Read the model definition and answer for the solid it produces. Units are mm, in the model's axes. A direction names the side the tool comes from. Give positions to 0.01 mm unless a question says otherwise; leave off trailing zeros. Order: outer loops, then holes, each group sorted by start corner. A loop starts at its lowest first (then second) coordinate and runs counter-clockwise, first axis right, second up.
Item 1: Given pin 1 Ø1.1 at (x, y) = (4, 0) entering from +Z; pin 2 Ø1.8 at (x, y) = (-6, 0.5) entering from -Z; pin 3 Ø2 at (x, y) = (0, 0.5) entering from +Z; pin 4 Ø4 at (x, y) = (0.5, 1) entering from +Z, each flat-ended and moving along its own axis, determine where each tip first touches the part or whether it passes through.
Item 2: Which of the six approach directions +Z, -Z, +X, -X, +Y, -Y give full straight-line access (tool end or side, diameter ignored) to faces 1 (the face through (-9.01, 0.7, 3.41)), 2 (the face through (-10.171, -1.045, -2.26)), 3 (the face through (-9.01, 0.7, 5.31))?
Item 3: A cutting plane is placed at A-A (z = -1). Write down the section's boundary in (x, y), plus the area to 3 significant figures.
Item 4: The mould has two halves that part along X. Classify faces 4 (the face through (-10.7, 0, 2)), 5 (the face through (11.4, 0, 0)), 6 (the face through (-0.2, -2.3, -3)): +X half, -X half, draft (parallel to the pull), parting line (faces both ways), or undercut.
Item 5: Find the intervals of material crossed by line 1 along X through (y, z) = (1.5, -0.5); line 2 along X through (y, z) = (0.5, -2.25); line 3 along Y through (x, z) = (-3, -1.25), in increasing order.
Item 6: A cutting plane is placed at B-B (x = -1.25). Write down the section's boundary in (y, z), plus the area to 3 significant figures.
Item 7: A cutting plane is placed at C-C (z = 0.5). Write down the section's boundary in (x, y), plus the area to 3 significant figures.
Item 8: A cutting plane is placed at D-D (x = 8). Write down the section's boundary in (y, z).
Autodesk Inventor part; units mm, degrees
ref_plane "Work Plane1" through (-8.1, 0, 4.8) normal (0, 0, 1) x (1, 0, 0)
ref_plane "Work Plane2" through (-11.4, 0, 3) normal (0, -1, 0) x (1, 0, 0)
ref_plane "YZ Plane" through (0, 0, 0) normal (1, 0, 0) x (0, 1, 0)
sketch "Sketch1" plane through (0, 0, 0) normal (0, 0, 1) x (1, 0, 0)
  line L0 (-11.4, -3.5) -> (11.4, -3.5)
  line L1 (11.4, -3.5) -> (11.4, 3.5)
  line L2 (11.4, 3.5) -> (-11.4, 3.5)
  line L3 (-11.4, 3.5) -> (-11.4, -3.5)
  line L4 (-11.4, -3.5) -> (11.4, 3.5) construction
  line L5 (11.4, -3.5) -> (-11.4, 3.5) construction
  point P0 (0, 0)
  dimension "d0" = 22.8
  dimension "d1" = 7
extrude "Extrusion1" add sketch "Sketch1" along normal mid plane 6
sketch "Sketch2" plane through (0, 0, 3) normal (0, 0, 1) x (1, 0, 0)
  line L0 (-5, 2.1) -> (-0.5, 2.1)
  line L1 (-0.5, 2.1) -> (-0.5, -2.1)
  line L2 (-0.5, -2.1) -> (-5, -2.1)
  line L3 (-5, -2.1) -> (-5, 2.1)
  line L4 (-5, 2.1) -> (-0.5, -2.1) construction
  line L5 (-0.5, 2.1) -> (-5, -2.1) construction
  line L6 (-11.4, 3.5) -> (-11.4, -3.5)
  line L7 (-2.75, 0) -> (-11.4, 0) construction
  point P0 (0, 0)
  dimension "d4" = 4.2
  dimension "d5" = 4.5
  dimension "d6" = 6.4
extrude "Extrusion2" cut sketch "Sketch2" against normal through all
sketch "Sketch3" plane through (0, 0, 3) normal (0, 0, 1) x (1, 0, 0)
  line L0 (-5, -2.1) -> (-5, 2.1)
  line L1 (-5, 2.1) -> (-0.5, 2.1)
  line L2 (-0.5, 2.1) -> (-0.5, -2.1)
  line L3 (-0.5, -2.1) -> (-5, -2.1)
  line L4 (-11.4, -3.5) -> (11.4, -3.5)
  line L5 (11.4, -3.5) -> (11.4, 3.5)
  line L6 (11.4, 3.5) -> (-11.4, 3.5)
  line L7 (-11.4, 3.5) -> (-11.4, -3.5)
  line L8 (-10.7, -2.6) -> (10.5, -2.6)
  line L9 (10.5, -2.6) -> (10.5, 2.6)
  line L10 (10.5, 2.6) -> (-10.7, 2.6)
  line L11 (-10.7, 2.6) -> (-10.7, -2.6)
  line L12 (-10.7, -2.6) -> (10.5, 2.6) construction
  line L13 (10.5, -2.6) -> (-10.7, 2.6) construction
  dimension "d11" = 0.7
  dimension "d12" = 0.9
  dimension "d13" = 5.2
  dimension "d14" = 21.2
extrude "Extrusion3" cut sketch "Sketch3" against normal blind 1.5 contours L11 L10 L9 L8
sketch "Sketch4" plane through (0, 0, -3) normal (0, 0, -1) x (-1, 0, 0)
  line L0 (-2.6, -2.1) -> (5, -2.1)
  line L1 (5, -2.1) -> (5, 2.1)
  line L2 (5, 2.1) -> (-2.6, 2.1)
  line L3 (-2.6, 2.1) -> (-2.6, -2.1)
  line L4 (-2.6, -2.1) -> (5, 2.1) construction
  line L5 (5, -2.1) -> (-2.6, 2.1) construction
  line L6 (5, 2.1) -> (5, -2.1)
  line L7 (5, -2.1) -> (0.5, -2.1)
  line L8 (0.5, -2.1) -> (0.5, 2.1)
  line L9 (0.5, 2.1) -> (5, 2.1)
  line L10 (-11.4, -3.5) -> (11.4, -3.5)
  line L11 (11.4, -3.5) -> (11.4, 3.5)
  line L12 (11.4, 3.5) -> (-11.4, 3.5)
  line L13 (-11.4, 3.5) -> (-11.4, -3.5)
  line L14 (0.5, 2.1) -> (5, 2.1)
  line L15 (5, -2.1) -> (0.5, -2.1)
  line L16 (5, 2.1) -> (5, -2.1)
  point P0 (0, 0)
  point P1 (1.2, 0)
  dimension "d17" = 14
extrude "Extrusion4" cut sketch "Sketch4" against normal blind 2.9 contours L3 L2 L8 L0 | L8 L2 L1 L0
sketch "Sketch5" plane through (0, 0, -3) normal (0, 0, -1) x (-1, 0, 0)
  line L0 (6.4, -2.1) -> (-6.5, -2.1)
  line L1 (-6.5, -2.1) -> (-6.5, 2.1)
  line L2 (-6.5, 2.1) -> (6.4, 2.1)
  line L3 (6.4, 2.1) -> (6.4, -2.1)
  line L4 (6.4, -2.1) -> (-6.5, 2.1) construction
  line L5 (-6.5, -2.1) -> (6.4, 2.1) construction
  line L6 (-2.6, 2.1) -> (5, 2.1)
  line L7 (5, -2.1) -> (-2.6, -2.1)
  line L8 (11.4, -3.5) -> (11.4, 3.5)
  point P0 (0, 0)
  point P1 (-0.05, 0)
  dimension "d20" = 12.9
  dimension "d21" = 5
extrude "Extrusion5" cut sketch "Sketch5" against normal blind 2.4
sketch "Sketch6" plane through (0, 0, -3) normal (0, 0, -1) x (-1, 0, 0)
  line L0 (-6.5, 2.1) -> (6.4, 2.1)
  line L1 (6.4, 2.1) -> (6.4, -2.1)
  line L2 (6.4, -2.1) -> (-6.5, -2.1)
  line L3 (-6.5, -2.1) -> (-6.5, 2.1)
  line L4 (-11.4, -3.5) -> (11.4, -3.5)
  line L5 (11.4, -3.5) -> (11.4, 3.5)
  line L6 (11.4, 3.5) -> (-11.4, 3.5)
  line L7 (-11.4, 3.5) -> (-11.4, -3.5)
  point P0 (0, 0)
hole "Hole1" at (-6.4, 2.1, -3) at (-6.4, -2.1, -3) at (6.5, -2.1, -3) at (6.5, 2.1, -3) direction (0, 0, 1) diameter 0.5 depth 2.4
sketch "Sketch7" plane through (0, 0, -3) normal (0, 0, -1) x (-1, 0, 0)
  line L0 (-11.4, -3.5) -> (11.4, -3.5)
  line L1 (11.4, -3.5) -> (11.4, 3.5)
  line L2 (11.4, 3.5) -> (-11.4, 3.5)
  line L3 (-11.4, 3.5) -> (-11.4, -3.5)
  arc A0 (-6.5, -1.85) -> (-6.25, -2.1) centre (-6.5, -2.1) ccw
  line L4 (-6.5, -1.85) -> (-6.5, 1.85)
  arc A1 (-6.25, 2.1) -> (-6.5, 1.85) centre (-6.5, 2.1) ccw
  line L5 (-6.25, 2.1) -> (6.15, 2.1)
  arc A2 (6.4, 1.85) -> (6.15, 2.1) centre (6.4, 2.1) ccw
  line L6 (6.4, 1.85) -> (6.4, -1.85)
  arc A3 (6.15, -2.1) -> (6.4, -1.85) centre (6.4, -2.1) ccw
  line L7 (6.15, -2.1) -> (-6.25, -2.1)
  line L8 (-6.5, -1.85) -> (-6.5, 1.85)
  line L9 (-11.4, 3.5) -> (-11.4, -3.5)
  line L10 (11.4, -3.5) -> (11.4, 3.5)
  line L11 (6.4, 1.85) -> (6.4, -1.85)
  arc A4 (9.4189, -0.0387) -> (6.4, 2.1) centre (6.4, -1.1) ccw
  arc A5 (8.4755, -0.3703) -> (6.4, 1.1) centre (6.4, -1.1) ccw
  arc A6 (9.4189, -0.0387) -> (11.4, -1.4422) centre (11.4, 0.6578) ccw
  arc A7 (8.4755, -0.3703) -> (11.4, -2.4422) centre (11.4, 0.6578) ccw
  line L12 (6.4, 1.1) -> (6.4, 2.1)
  line L13 (11.4, -2.4422) -> (11.4, -1.4422)
  line L14 (11.4, 3.5) -> (11.4, -3.5)
  point P0 (0, 0)
  dimension "d36" = 1
  dimension "d37" = 2.2
  dimension "d38" = 2.1
extrude "Extrusion7" cut sketch "Sketch7" against normal blind 1.5 contours A7 A5 L6 A2 A4 A6 L1 | A2 L12 A4
sketch "Sketch8" plane through (0, 0, -0.6) normal (0, 0, -1) x (-1, 0, 0)
  line L0 (11.4, 3.5) -> (-11.4, 3.5)
  line L1 (11.4, -3.5) -> (11.4, -2.4422)
  point P0 (0, 0)
  point P1 (-4, 0)
  dimension "d41" = 3.5
  dimension "d42" = 15.4
hole "Hole2" at (4, 0, -0.6) direction (0, 0, 1) diameter 1.181 end through all
sketch "Sketch9" plane through (0, 0, 1.5) normal (0, 0, 1) x (1, 0, 0)
  circle A0 centre (-8.1, 0) radius 1.15
  circle A1 centre (8, 0) radius 1.15
  line L0 (-8.1, 0) -> (8, 0) construction
  line L1 (11.4, 3.5) -> (-11.4, 3.5)
  line L2 (-11.4, 3.5) -> (-11.4, -3.5)
  point P0 (0, 0)
  dimension "d50" = 3.5
  dimension "d51" = 16.1
  dimension "d52" = 3.3
  dimension "d53" = 2.3
extrude "Extrusion8" add sketch "Sketch9" along normal blind 4.5
chamfer "Chamfer1" distance 0.3 angle 45 2 edges at (-9.25, 0, 6) (6.85, 0, 6)
ref_plane "Work Plane1" through (-8.1, 0, 4.8) normal (0, 0, 1) x (1, 0, 0)
sketch "Sketch10" plane through (-8.1, 0, 4.8) normal (0, 0, 1) x (1, 0, 0)
  circle A0 centre (0, 0) radius 1.15
  circle A1 centre (16.1, 0) radius 1.15
  circle A2 centre (0, 0) radius 1.2
  circle A3 centre (16.1, 0) radius 1.2
  point P0 (8.1, 0)
  dimension "d60" = 2.4
  dimension "d61" = 2.4
extrude "Extrusion9" add sketch "Sketch10" against normal blind 0.2
ref_plane "Work Plane2" through (-11.4, 0, 3) normal (0, -1, 0) x (1, 0, 0)
sketch "Sketch11" plane through (-11.4, 0, 3) normal (0, -1, 0) x (1, 0, 0)
  line L0 (4.45, 2.7) -> (2.15, 2.7)
  line L1 (4.45, 1.8) -> (2.15, 1.8)
  line L2 (2.1, 1.6) -> (4.5, 1.6)
  line L3 (2.1, 1.8) -> (4.5, 1.8)
  line L4 (2.15, 1.6) -> (4.45, 1.6)
  line L5 (2.15, -1.5) -> (4.45, -1.5)
  line L6 (20.55, 2.7) -> (18.25, 2.7)
  line L7 (20.55, 1.8) -> (18.25, 1.8)
  line L8 (18.2, 1.6) -> (20.6, 1.6)
  line L9 (18.2, 1.8) -> (20.6, 1.8)
  line L10 (18.25, 1.6) -> (20.55, 1.6)
  line L11 (18.25, -1.5) -> (20.55, -1.5)
  line L12 (2.1, 1.8) -> (4.5, 1.8)
  line L13 (2.1, 1.8) -> (2.15, 1.9374)
  line L14 (2.1, 1.6) -> (2.15, 1.55)
  line L15 (2.15, -1.5) -> (2.15, 1.6)
  line L16 (2.15, 1.8) -> (2.15, 2.7)
  line L17 (2.15, 1.9374) -> (2.15, 1.8)
  line L18 (2.1, 1.8) -> (2.15, 1.8)
  line L19 (2.15, 1.55) -> (2.15, 1.6)
  line L20 (2.1, 1.6) -> (4.5, 1.6)
  line L21 (2.1, 1.6) -> (2.15, 1.6)
  line L22 (2.45, 3) -> (4.15, 3)
  line L23 (3.3, 3) -> (3.3, 1.6)
  line L24 (2.15, 1.6) -> (4.45, 1.6)
  point P0 (11.4, -3)
  dimension "d68" = 20
  dimension "d69" = 45
revolve "Revolution1" add sketch "Sketch11" angle 360 about axis through (-8.1, 0, 6) along (0, 0, -1) contours L15 L14 L2 | L16 L3 L13
sketch "Sketch12" plane through (-11.4, 0, 3) normal (0, -1, 0) x (1, 0, 0)
  line L0 (18.25, 1.8) -> (18.25, 2.7)
  line L1 (18.2, 1.8) -> (20.6, 1.8)
  line L2 (18.2, 1.8) -> (18.2, 1.6)
  line L3 (18.25, -1.5) -> (18.25, 1.6)
  line L4 (18.2, 1.6) -> (20.6, 1.6)
  line L5 (20.6, 1.8) -> (20.6, 1.6)
  line L6 (20.55, 1.8) -> (20.55, 2.7)
  line L7 (20.55, -1.5) -> (20.55, 1.6)
  line L8 (18.2, 1.8) -> (18.25, 1.9374)
  line L9 (20.55, 1.8) -> (18.25, 1.8)
  line L10 (18.25, 1.8) -> (18.25, 1.9374)
  line L11 (18.25, 1.8) -> (18.2, 1.8)
  line L12 (18.25, 1.55) -> (18.2, 1.6)
  line L13 (18.25, 1.6) -> (20.55, 1.6)
  line L14 (18.25, 1.6) -> (18.2, 1.6)
  line L15 (18.25, 1.6) -> (18.25, 1.55)
  line L16 (18.55, 3) -> (20.25, 3)
  line L17 (19.4, 3) -> (19.4, 1.6)
  point P0 (11.4, -3)
  dimension "d71" = 70
  dimension "d72" = 45
revolve "Revolution2" add sketch "Sketch12" angle 360 about axis through (8, 0, 6) along (0, 0, -1) contours L1 L8 L0 | L4 L3 L12
fillet "Fillet1" radius 0.8 2 edges at (-9.25, 0, 1.5) (6.85, 0, 1.5)
properties part number "sipmHolder" material "ABS Plastic"
Response values:
1. pin 1: passes through
1. pin 2: stops at z = -3
1. pin 3: stops at z = 1.5
1. pin 4: stops at z = 3
2. face 1: none
2. face 2: -Z
2. face 3: +Z
3. outline: (-11.4, -3.5) - (11.4, -3.5) - (11.4, 3.5) - (-11.4, 3.5) - close; hole (-6.4, -1.85) arc R0.25 ccw (long way) to (-6.15, -2.1) - (6.25, -2.1) arc R0.25 ccw (long way) to (6.5, -1.85) - (6.5, 1.85) arc R0.25 ccw (long way) to (6.25, 2.1) - (-6.15, 2.1) arc R0.25 ccw (long way) to (-6.4, 1.85) - close
3. area: 105 mm2
4. face 4: undercut
4. face 5: +X half
4. face 6: draft
5. line 1: x = -11.4 to -5, 2.6 to 11.4
5. line 2: x = -11.4 to -9.17, -7.91 to -6.4, 6.5 to 11.4
5. line 3: y = -3.5 to -2.1, 2.1 to 3.5
6. outline: (-3.5, -3) - (-2.1, -3) - (-2.1, 1.5) - (-2.6, 1.5) - (-2.6, 3) - (-3.5, 3) - close; (2.1, -3) - (3.5, -3) - (3.5, 3) - (2.6, 3) - (2.6, 1.5) - (2.1, 1.5) - close
6. area: 15.3 mm2
7. outline: (-11.4, -3.5) - (11.4, -3.5) - (11.4, 3.5) - (-11.4, 3.5) - close; hole (-5, -2.1) - (-0.5, -2.1) - (-0.5, 2.1) - (-5, 2.1) - close; hole circle Ø1.18 at (4, 0)
7. area: 140 mm2
8. outline: (-3.5, -3) - (3.5, -3) - (3.5, 3) - (2.6, 3) - (2.6, 1.5) - (1.95, 1.5) arc R0.8 cw to (1.15, 2.3) - (1.15, 4.55) - (1.2, 4.6) - (1.2, 4.8) - (1.15, 4.94) - (1.15, 5.7) - (0.85, 6) - (-0.85, 6) - (-1.15, 5.7) - (-1.15, 4.94) - (-1.2, 4.8) - (-1.2, 4.6) - (-1.15, 4.55) - (-1.15, 2.3) arc R0.8 cw to (-1.95, 1.5) - (-2.6, 1.5) - (-2.6, 3) - (-3.5, 3) - close
